Read the model definition and answer for the solid it produces. Units are mm, in the model's axes. A direction names the side the tool comes from. Coordinates: 2 decimals unless noted, no trailing zeros. Write each loop counter-clockwise with the first axis right and the second up, starting at its lowest first coordinate (ties: lowest second). Pieces come first, ordered by that corner, then holes. Notation, with made-up numbers: (-1, 80) - (8, 80) arc R20 ccw to (8, 101) - close; hole circle Ø5 at (89.25, 57). An arc over 180 degrees is marked (long way). Use a Markdown table: item, result.
from build123d import *

# Parameters (mm, degrees)
SKETCH1_W           = 30
SKETCH1_H           = 30
BOSS_EXTRUDE1_DEPTH = 22
CUT_EXTRUDE1_DEPTH  = 48.791212581


with BuildPart() as part:
    # Sketch1 → Boss-Extrude1 (new body)
    with BuildSketch(Plane(origin=(0, 0, 0), x_dir=(1, 0, 0), z_dir=(0, 1, 0))):
        with Locations((15, 15)):
            Rectangle(SKETCH1_W, SKETCH1_H)
    extrude(amount=BOSS_EXTRUDE1_DEPTH)

    # Sketch2 → Cut-Extrude1 (cut, through all)
    with BuildSketch(Plane.XY):
        Polygon((7.574494777, 18.379095815), (11.195398962, 22), (0, 22), (0, 2.847414058), (1.559595822, 4.407009879), (1.559595822, 18.379095815), align=None)
        Polygon((30, 22), (18.804601038, 22), (22.425505223, 18.379095815), (28.440404178, 18.379095815), (28.440404178, 4.407009879), (30, 2.847414058), align=None)
        with BuildLine():
            ThreePointArc((19, 11), (17.828427125, 13.828427125), (15, 15))
            Line((15, 15), (15, 7))
            ThreePointArc((15, 7), (17.828427125, 8.171572875), (19, 11))
        make_face()
        with BuildLine():
            Line((15, 7), (15, 15))
            ThreePointArc((15, 15), (11, 11), (15, 7))
        make_face()
    extrude(amount=-CUT_EXTRUDE1_DEPTH, mode=Mode.SUBTRACT)


solid = part.part
(1) Each of these flat-tipped pins is pushed along its axis until it touches: P1, Ø3, axis at x = 3.5, z = -17.5, coming from the +Y side; P2, Ø5, axis at x = 22, z = -16, coming from the +Y side; P3, Ø11, axis at y = 9.5, z = -20.5, coming from the -X side. Where does it stop, or does it pass through?
Report:
| item | result |
|---|---|
| P1 | stops at y = 18.38 |
| P2 | stops at y = 21.3 |
| P3 | stops at x = 1.15 |
(2) A cutting plane is placed at A-A, the plane z = -11. Write down the section's boundary in (x, y), and give its area (3 significant figures).
Report:
| item | result |
|---|---|
| outline | (0, 0) - (30, 0) - (30, 2.85) - (28.44, 4.41) - (28.44, 18.38) - (22.43, 18.38) - (18.8, 22) - (11.2, 22) - (7.57, 18.38) - (1.56, 18.38) - (1.56, 4.41) - (0, 2.85) - close; hole circle Ø8 at (15, 11) |
| area | 496 mm² |
(3) A cutting plane is placed at D-D, the plane y = 20.25. Write down the section's boundary in (x, z), and give its area (3 significant figures).
Report:
| item | result |
|---|---|
| outline | (9.45, -30) - (20.55, -30) - (20.55, 0) - (9.45, 0) - close |
| area | 333 mm² |
(4) A cutting plane is placed at C-C, the plane x = 24. Write down the section's boundary in (y, z).
Report:
| item | result |
|---|---|
| outline | (0, -30) - (18.38, -30) - (18.38, 0) - (0, 0) - close |
(5) Straight lines are drawn through the part: L1, parallel to Y at x = 12, z = -3.5; L2, parallel to X at y = 5.75, z = -5; L3, parallel to Y at x = 18.5, z = -11. For each, find the intervals that lie inside material, in ascending order.
Report:
| item | result |
|---|---|
| L1 | y = 0 to 8.35, 13.65 to 22 |
| L2 | x = 1.56 to 28.44 |
| L3 | y = 0 to 9.06, 12.94 to 22 |
(6) For faces 1 (the flat face through (0, 1, -15)), 2 (the flat face through (28.44, 11, -15)), 3 (the flat face through (1.56, 11, -15)), determine the directions among +Z, -Z, +X, -X, +Y, -Y from which every point of the face is accessible in a straight line to the end or side of a thin tool.
Report:
| item | result |
|---|---|
| face 1 | +Z, -Z, -X, +Y, -Y |
| face 2 | +Z, -Z, +X, +Y |
| face 3 | +Z, -Z, -X, +Y |
(7) A cutting plane is placed at B-B, the plane x = 11.75. Write down the section's boundary in (y, z).
Report:
| item | result |
|---|---|
| outline | (0, -30) - (8.67, -30) - (8.67, 0) - (0, 0) - close; (13.33, -30) - (22, -30) - (22, 0) - (13.33, 0) - close |
